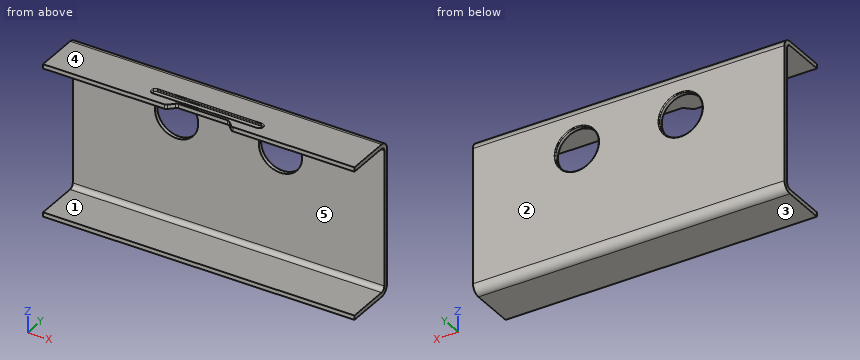
```python
from build123d import *

# Parameters (mm, degrees)
SKETCH1_W           = 18
SKETCH1_H           = 8.8
BOSS_EXTRUDE1_DEPTH = 3
SKETCH2_R           = 1.25
CUT_EXTRUDE1_DEPTH  = 3
FILLET1_R           = 0.5
CUT_EXTRUDE2_DEPTH  = 23
SKETCH4_W           = 4
SKETCH4_H           = 1.424515237
CUT_EXTRUDE3_DEPTH  = 2
CHAMFER1_SIZE       = 0.5
CUT_EXTRUDE4_DEPTH  = 0.1
FILLET2_R           = 0.05
FILLET3_R           = 0.2
FILLET4_R           = 0.05


# Some blends are built 0.0001 mm under size
with BuildPart() as part:
    # Sketch1 → Boss-Extrude1 (new body)
    with BuildSketch(Plane(origin=(0, 0, 0), x_dir=(1, 0, 0), z_dir=(0, 1, 0))):
        Rectangle(SKETCH1_W, SKETCH1_H)
    extrude(amount=BOSS_EXTRUDE1_DEPTH)

    # Sketch2 → Cut-Extrude1 (cut)
    with BuildSketch(Plane(origin=(0, 3, 0), x_dir=(1, 0, 0), z_dir=(0, 1, 0))):
        with Locations(Location((-3, -1.9, 0), (0, 0, 270))):
            Circle(SKETCH2_R)
        with Locations(Location((3, -1.9, 0), (0, 0, 270))):
            Circle(SKETCH2_R)
    extrude(amount=-CUT_EXTRUDE1_DEPTH, mode=Mode.SUBTRACT)

    # Fillet1
    fillet1_edges = [part.edges().sort_by_distance(p)[0] for p in [
        (0, 3, -4.4),
        (0, 3, 4.4),
    ]]
    fillet(fillet1_edges, radius=FILLET1_R)

    # Sketch3 → Cut-Extrude2 (cut)
    with BuildSketch(Plane.ZY.offset(9)):
        with BuildLine():
            Line((-4.15, 0.25), (-4.15, -7.258391717))
            Line((-4.15, -7.258391717), (4.15, -7.258391717))
            Line((4.15, -7.258391717), (4.15, 0.25))
            Line((4.15, 0.25), (4.15, 2.5))
            ThreePointArc((4.15, 2.5), (4.076776695, 2.676776695), (3.9, 2.75))
            Line((3.9, 2.75), (-3.9, 2.75))
            ThreePointArc((-3.9, 2.75), (-4.076776695, 2.676776695), (-4.15, 2.5))
            Line((-4.15, 2.5), (-4.15, 0.25))
        make_face()
    extrude(amount=-CUT_EXTRUDE2_DEPTH, mode=Mode.SUBTRACT)

    # Sketch4 → Cut-Extrude3 (cut)
    with BuildSketch(Plane.XY.offset(4.4)):
        with Locations((0, -0.312257619)):
            Rectangle(SKETCH4_W, SKETCH4_H)
    extrude(amount=-CUT_EXTRUDE3_DEPTH, mode=Mode.SUBTRACT)

    # Chamfer1
    # the kernel refuses this chamfer: 0.5 mm, written as the material it adds along each edge
    with BuildSketch(Plane(origin=(2, 0.4, 4.4), x_dir=(0.027495876610586487, -0.9996219169112968, 0), z_dir=(0, 0, -1))) as chamfer1_piece_1_section:
        Polygon((CHAMFER1_SIZE * 0.999621916911, CHAMFER1_SIZE * 0.0274958766106), (-CHAMFER1_SIZE * 0.0274958766106, CHAMFER1_SIZE * 0.999621916911), (0, 0), align=None)
    chamfer1_piece_1 = extrude(amount=0.25, mode=Mode.PRIVATE)
    chamfer1_piece_1 = split(chamfer1_piece_1, bisect_by=Plane(origin=(1.827140794, 0, 4.275), z_dir=(0, 1, 0)), keep=Keep.TOP, mode=Mode.PRIVATE)
    add(chamfer1_piece_1)
    with BuildSketch(Plane(origin=(-2, 0.4, 4.4), x_dir=(0.9996219169112968, 0.02749587661058639, 0), z_dir=(0, 0, -1))) as chamfer1_piece_2_section:
        Polygon((CHAMFER1_SIZE * 0.999621916911, CHAMFER1_SIZE * 0.0274958766106), (-CHAMFER1_SIZE * 0.0274958766106, CHAMFER1_SIZE * 0.999621916911), (0, 0), align=None)
    chamfer1_piece_2 = extrude(amount=0.25, mode=Mode.PRIVATE)
    chamfer1_piece_2 = split(chamfer1_piece_2, bisect_by=Plane(origin=(-1.827140794, 0, 4.275), z_dir=(0, 1, 0)), keep=Keep.TOP, mode=Mode.PRIVATE)
    add(chamfer1_piece_2)

    # Sketch5 → Cut-Extrude4 (cut)
    with BuildSketch(Plane.XY.offset(4.4)):
        with BuildLine():
            Line((-3, 1), (3, 1))
            ThreePointArc((3, 1), (3.2, 0.8), (3, 0.6))
            Line((3, 0.6), (-3, 0.6))
            ThreePointArc((-3, 0.6), (-3.2, 0.8), (-3, 1))
        make_face()
    extrude(amount=-CUT_EXTRUDE4_DEPTH, mode=Mode.SUBTRACT)

    # Fillet2
    fillet2_edges = [part.edges().sort_by_distance(p)[0] for p in [
        (3.2, 0.8, 4.4),
        (0, 0.6, 4.4),
        (-3.2, 0.8, 4.4),
        (0, 1, 4.3),
        (3.2, 0.8, 4.3),
        (0, 0.6, 4.3),
        (-3.2, 0.8, 4.3),
        (0, 1, 4.4),
    ]]
    fillet(fillet2_edges, radius=FILLET2_R - 0.0001)  # a hair under: the kernel refuses the full size

    # Fillet3
    fillet3_edges = [part.edges().sort_by_distance(p)[0] for p in [
        (-1.5, 0.4, 4.275),
        (1.5, 0.4, 4.275),
        (1.9, 0, 4.275),
        (-1.9, 0, 4.275),
    ]]
    fillet(fillet3_edges, radius=FILLET3_R)

    # Fillet4
    fillet4_edges = [part.edges().sort_by_distance(p)[0] for p in [
        (-3, 3, 0.65),
        (3, 3, 0.65),
    ]]
    fillet(fillet4_edges, radius=FILLET4_R)


solid = part.part
```
Part model, mm, in its own coordinate system. Face numbers are marked on the shaded views. A direction names the side the tool comes from. Round coordinates to 2 decimals unless told otherwise and drop trailing zeros. Write each loop counter-clockwise with the first axis right and the second up, starting at its lowest first coordinate (ties: lowest second). Pieces come first, ordered by that corner, then holes. Notation, with made-up numbers: (36.5, 78) -> (40.5, 78) arc R26 cw to (40.5, 93) -> close; hole circle Ø11 at (68, 50.25). An arc over 180 degrees is marked (long way). Return JSON: item names as keys, results as strings. Group by question number.
Q1. Saw through at B-B on z = 1.9. Write the cut outline in (x, y).
Q2. Saw through at C-C on x = -6.25. Write the cut outline in (y, z).
Q3. Probe L1, parallel to X at y = 2.9, z = 1.9; L2, parallel to Z at x = 2, y = 0.2; L3, parallel to Y at x = -4.5, z = -2.5. List the from-to ranges inside material, lowest first. Write a range as [from, to].
Q4. Mould opens along Z. For the marked faces 1, 2 and 3 say: pulls with the +Z half, pulls with the -Z half, needs draft (parallel to the pull), parting line crosses it, or undercut.
Q5. Saw through at D-D on z = -1.5. Write the cut outline in (x, y).
Q6. Which spindle directions (+Z, -Z, +X, -X, +Y, -Y) get a long thin tool onto all of the face, cutting with end or side? Do the marked faces 4 and 5. Say none if no direction does.
Q7. Saw through at A-A on y = 2.2. Write the cut outline in (x, z).
Q8. Pin check, flat tips, straight feed: pin 1 (3 mm diameter, centred on x = 2, z = -2.5, fed in from -Y); pin 2 (4 mm diameter, centred on x = 3.5, z = 0.5, fed in from -Y). Stop position of each tip, or through.
Answer:
{
 "1": {"outline": "(-9, 2.75) -> (-4.25, 2.75) -> (-4.25, 2.95) arc R0.05 ccw to (-4.3, 3) -> (-9, 3) -> close; (-1.75, 2.75) -> (1.75, 2.75) -> (1.75, 2.95) arc R0.05 ccw to (1.7, 3) -> (-1.7, 3) arc R0.05 ccw to (-1.75, 2.95) -> close; (4.25, 2.75) -> (9, 2.75) -> (9, 3) -> (4.3, 3) arc R0.05 ccw to (4.25, 2.95) -> close"},
 "2": {"outline": "(0, -4.4) -> (2.5, -4.4) arc R0.5 ccw to (3, -3.9) -> (3, 3.9) arc R0.5 ccw to (2.5, 4.4) -> (0, 4.4) -> (0, 4.15) -> (2.5, 4.15) arc R0.25 cw to (2.75, 3.9) -> (2.75, -3.9) arc R0.25 cw to (2.5, -4.15) -> (0, -4.15) -> close"},
 "3": {"L1": "[-9, -4.25], [-1.75, 1.75], [4.25, 9]", "L2": "[-4.4, -4.15], [4.15, 4.4]", "L3": "[2.75, 3]"},
 "4": {"face 1": "undercut", "face 2": "needs draft", "face 3": "pulls with the -Z half"},
 "5": {"outline": "(-9, 2.75) -> (9, 2.75) -> (9, 3) -> (-9, 3) -> close"},
 "6": {"face 4": "+Z, +X, -X, +Y, -Y", "face 5": "+X, -X, -Y"},
 "7": {"outline": "(-9, -4.4) -> (9, -4.4) -> (9, -4.15) -> (-9, -4.15) -> close; (-9, 4.15) -> (9, 4.15) -> (9, 4.4) -> (-9, 4.4) -> close"},
 "8": {"pin 1": "y = 2.73", "pin 2": "y = 2.75"}
}
